The listing builds one solid part. Answer for the finished solid, in the listing's coordinates (mm). A direction names the side the tool comes from. Coordinates: 2 decimals unless noted, no trailing zeros. Order: outer loops, then holes, each group sorted by start corner. A loop starts at its lowest first (then second) coordinate and runs counter-clockwise, first axis right, second up.
```python
from build123d import *

# Parameters (mm, degrees)
SKETCH1_R               = 8
BOSS_EXTRUDE1_DEPTH     = 117
SKETCH2_W               = 66
SKETCH2_H               = 34
CUT_EXTRUDE1_DEPTH      = 31
CUT_EXTRUDE1_DEPTH_BACK = 31
CUT_EXTRUDE2_DEPTH      = 22


with BuildPart() as part:
    # Sketch1 → Boss-Extrude1 (new body)
    with BuildSketch(Plane.XY):
        Polygon((30, 19), (-30, 19), (-30, -41), (-21, -41), (-21, -31), (-13, -31), (-13, -15), (13, -15), (13, -31), (21, -31), (21, -41), (30, -41), align=None)
        Circle(SKETCH1_R, mode=Mode.SUBTRACT)
    extrude(amount=BOSS_EXTRUDE1_DEPTH)

    # Sketch2 → Cut-Extrude1 (cut, two sides)
    with BuildSketch(Plane(origin=(0, 0, 0), x_dir=(0, 0, -1), z_dir=(1, 0, 0))) as cut_extrude1_sk:
        Polygon((-117, 3), (-101, 19), (-117, 19), align=None)
        with Locations((-55, 2)):
            Rectangle(SKETCH2_W, SKETCH2_H)
    extrude(amount=CUT_EXTRUDE1_DEPTH, mode=Mode.SUBTRACT)
    extrude(cut_extrude1_sk.sketch, amount=-CUT_EXTRUDE1_DEPTH_BACK, mode=Mode.SUBTRACT)

    # Sketch1<3> → Cut-Extrude2 (cut)
    with BuildSketch(Plane.XY):
        Polygon((30, 3), (30, 19), (14, 19), align=None)
        Polygon((-30, 3), (-14, 19), (-30, 19), align=None)
    extrude(amount=CUT_EXTRUDE2_DEPTH, mode=Mode.SUBTRACT)


solid = part.part
```
1) For faces 4 (the flat face through (-26, -41, 58)), 5 (the flat face through (-17, -31, 58)), 6 (the flat face through (21, -15, 55)), determine the directions among +Z, -Z, +X, -X, +Y, -Y from which every point of the face is accessible in a straight line to the end or side of a thin tool.
2) A cutting plane is placed at C-C, the plane x = 0. Write down the section's boundary in (y, z), plus the area to 4 significant figures.
3) A cutting plane is placed at B-B, the plane y = 0. Write down the section's boundary in (x, z), plus the area to 3 significant figures.
4) The mould has two halves that part along X. Classify faces 1 (the flat face through (0, -14, 117)), 2 (the flat face through (-22, 11, 11)), 3 (the flat face through (0, -15, 102)): released by +X, released by -X, zero draft, split by the parting line, or undercut.
5) A cutting plane is placed at D-D, the plane z = 9. Write down the section's boundary in (x, y), plus the area to 3 significant figures.
6) Each of these flat-tipped pins is pushed along its axis until it touches: P1, Ø18.5, axis at x = 25.5, z = 62.5, coming from the +Y side; P2, Ø2, axis at x = 10.5, y = -20, coming from the -Z side; P3, Ø1.5, axis at x = -23.5, y = 12.5, coming from the +Z side; P4, Ø5, axis at x = -11.5, z = 89, coming from the -Y side. Where does it stop, or does it pass through?
7) Straight lines are drawn through the part: probe 1 along X at (y, z) = (0, 5.5); probe 2 along Y at (x, z) = (0, 16.75); probe 3 along Z at (x, y) = (-11.5, -13). For each, find the intervals that lie inside material, in ascending order.
8) A cutting plane is placed at A-A, the plane z = 55. Write down the section's boundary in (x, y).
Working result:
1. face 4: +Z, -Z, +X, -X, -Y
1. face 5: +Z, -Z, -Y
1. face 6: +X, -X, +Y
2. outline: (-15, 0) - (-8, 0) - (-8, 22) - (-15, 22) - close; (-15, 88) - (-8, 88) - (-8, 117) - (-15, 117) - close; (8, 0) - (19, 0) - (19, 22) - (8, 22) - close; (8, 88) - (19, 88) - (19, 101) - (8, 112) - close
2. area: 802.5 mm2
3. outline: (-30, 0) - (-8, 0) - (-8, 22) - (-30, 22) - close; (-30, 88) - (-8, 88) - (-8, 117) - (-30, 117) - close; (8, 0) - (30, 0) - (30, 22) - (8, 22) - close; (8, 88) - (30, 88) - (30, 117) - (8, 117) - close
3. area: 2,240 mm2
4. face 1: zero draft
4. face 2: released by -X
4. face 3: undercut
5. outline: (-30, -41) - (-21, -41) - (-21, -31) - (-13, -31) - (-13, -15) - (13, -15) - (13, -31) - (21, -31) - (21, -41) - (30, -41) - (30, 3) - (14, 19) - (-14, 19) - (-30, 3) - close; hole circle Ø16 at (0, 0)
5. area: 2,310 mm2
6. P1: stops at y = -15
6. P2: passes through
6. P3: stops at z = 108.25
6. P4: stops at y = -31
7. probe 1: x = -30 to -8, 8 to 30
7. probe 2: y = -15 to -8, 8 to 19
7. probe 3: z = 0 to 22, 88 to 117
8. outline: (-30, -41) - (-21, -41) - (-21, -31) - (-13, -31) - (-13, -15) - (-30, -15) - close; (13, -31) - (21, -31) - (21, -41) - (30, -41) - (30, -15) - (13, -15) - close
